Geometry check sheet. Reference: drawing and pictorial views, mm from the part's lowest x, y, z. Coordinates: 2 decimals unless noted, no trailing zeros. Write each loop counter-clockwise with the first axis right and the second up, starting at its lowest first coordinate (ties: lowest second). Pieces come first, ordered by that corner, then holes. Notation, with made-up numbers: (79, 50) - (85, 50) arc R27 cw to (85, 83) - close; hole circle Ø1 at (-9, 22). An arc over 180 degrees is marked (long way). Use one line per item in the form item = value. Start each with the question number.
(1) Sectioned sample at D-D (y = 18.5). Record the cut outline in (x, z).
(2) Sectioned sample at C-C (z = 7.5). Record the cut outline in (x, y).
(3) Sectioned sample at B-B (x = 3.25). Record the cut outline in (y, z).
(4) Material ranges on line 1 (Y direction, x = 11, z = 9.5); line 2 (X direction, y = 10.5, z = 7.25); line 3 (X direction, y = 10.75, z = 8.75), recorded low to high. Write a range as [from, to].
(5) Gauge pin test, flat ends, axial feed: pin 1 Ø1.6 at (x, y) = (19, 11) entering from -Z; pin 2 Ø5 at (y, z) = (14, 7) entering from +X; pin 3 Ø2 at (x, z) = (2.5, 4.5) entering from +Y; pin 4 Ø4 at (y, z) = (10, 4.5) entering from -X. Record the tip position at first contact, or that the pin passes through.
(6) Sectioned sample at A-A (y = 11). Record the cut outline in (x, z).
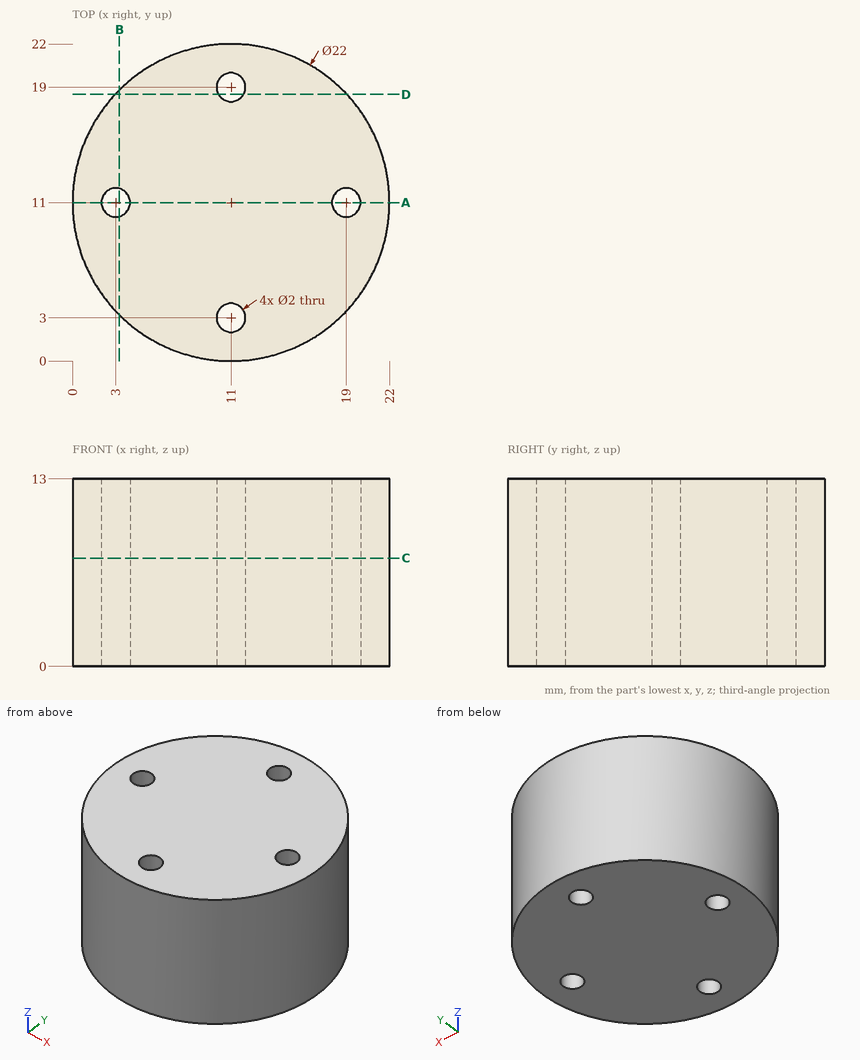
Answers below:
q1.outline = (2.95, 0) - (10.13, 0) - (10.13, 13) - (2.95, 13) - close; (11.87, 0) - (19.05, 0) - (19.05, 13) - (11.87, 13) - close
q2.outline = circle Ø22 at (11, 11); hole circle Ø2 at (3, 11); hole circle Ø2 at (11, 3); hole circle Ø2 at (11, 19); hole circle Ø2 at (19, 11)
q3.outline = (3.19, 0) - (10.03, 0) - (10.03, 13) - (3.19, 13) - close; (11.97, 0) - (18.81, 0) - (18.81, 13) - (11.97, 13) - close
q4.line_1 = [0, 2], [4, 18], [20, 22]
q4.line_2 = [0.01, 2.13], [3.87, 18.13], [19.87, 21.99]
q4.line_3 = [0, 2.03], [3.97, 18.03], [19.97, 22]
q5.pin_1 = through
q5.pin_2 = 21.99
q5.pin_3 = 19.05
q5.pin_4 = 0
q6.outline = (0, 0) - (2, 0) - (2, 13) - (0, 13) - close; (4, 0) - (18, 0) - (18, 13) - (4, 13) - close; (20, 0) - (22, 0) - (22, 13) - (20, 13) - close
